Verification items for the finished model (mm, model axes). A direction names the side the tool comes from. Coordinates: 2 decimals unless noted, no trailing zeros. Write each loop counter-clockwise with the first axis right and the second up, starting at its lowest first coordinate (ties: lowest second). Pieces come first, ordered by that corner, then holes.
```python
from build123d import *

# Parameters (mm, degrees)
SKETCH1_R           = 63.5
SKETCH1_R_2         = 3.96875
BOSS_EXTRUDE1_DEPTH = 12.7
SKETCH2_R           = 53.34
SKETCH2_R_2         = 12.7
CUT_EXTRUDE1_DEPTH  = 10.16


with BuildPart() as part:
    # Sketch1 → Boss-Extrude1 (new body, symmetric)
    with BuildSketch(Plane.XY):
        Circle(SKETCH1_R)
        Circle(SKETCH1_R_2, mode=Mode.SUBTRACT)
    extrude(amount=BOSS_EXTRUDE1_DEPTH, both=True)

    # Sketch2 → Cut-Extrude1 (cut)
    with BuildSketch(Plane.XY.offset(12.7)):
        Circle(SKETCH2_R)
        Circle(SKETCH2_R_2, mode=Mode.SUBTRACT)
    cut_extrude1 = extrude(amount=-CUT_EXTRUDE1_DEPTH, mode=Mode.SUBTRACT)

    # Mirror1: Cut-Extrude1 across plane
    add(cut_extrude1.mirror(Plane.XY), mode=Mode.SUBTRACT)


solid = part.part
```
1. Sectioned sample at C-C, the plane z = -6.5. Record the boundary of the cut face in (x, y), and give its area (3 significant figures).
2. Draft check along X on faces 4 (the cylindrical face through (-13.77, -61.99, 0.18)), 5 (the cylindrical face through (-0.86, -3.874, -0.178)), 6 (the flat face through (3, 3, 12.7)), 7 (the cylindrical face through (-2.75, -12.4, 7.69)). Enter one of: pulls with the +X half, pulls with the -X half, needs draft (parallel to the pull), parting line crosses it, or undercut.
3. Tool access check on faces 1 (the cylindrical face through (-6.944, 52.886, 7.691)), 2 (the cylindrical face through (-6.944, 52.886, -7.691)), 3 (the flat face through (-14, 52, -12.7)). Record the directions out of +Z, -Z, +X, -X, +Y, -Y that give a thin tool (end or side, any length) a straight path to the whole face; none if there is none.
4. Gauge pin test, flat ends, axial feed: P1, Ø5, axis at x = -33, y = -35, coming from the +Z side; P2, Ø2, axis at y = -10, z = -7, coming from the -X side; P3, Ø2, axis at x = 19.5, z = 8.5, coming from the +Y side. Record the tip position at first contact, or that the pin passes through.
5. Sectioned sample at D-D, the plane y = 25. Record the boundary of the cut face in (x, z).
6. Sectioned sample at A-A, the plane y = 0. Record the boundary of the cut face in (x, z), and give its area (3 significant figures).
7. Material ranges on L1, parallel to Y at x = 0, z = 4; L2, parallel to Z at x = 29, y = -26; L3, parallel to X at y = -6.5, z = 11, recorded low to high.
Outcome:
1. outline: circle Ø127 at (0, 0); circle Ø25.4 at (0, 0); hole circle Ø106.68 at (0, 0); hole circle Ø7.94 at (0, 0)
1. area: 4,190 mm2
2. face 4: parting line crosses it
2. face 5: undercut
2. face 6: needs draft
2. face 7: undercut
3. face 1: +Z
3. face 2: -Z
3. face 3: -Z, +X, -X, +Y, -Y
4. P1: stops at z = 2.54
4. P2: stops at x = -62.86
4. P3: stops at y = 60.75
5. outline: (-58.37, -12.7) - (-47.12, -12.7) - (-47.12, -2.54) - (47.12, -2.54) - (47.12, -12.7) - (58.37, -12.7) - (58.37, 12.7) - (47.12, 12.7) - (47.12, 2.54) - (-47.12, 2.54) - (-47.12, 12.7) - (-58.37, 12.7) - close
6. outline: (-63.5, -12.7) - (-53.34, -12.7) - (-53.34, -2.54) - (-12.7, -2.54) - (-12.7, -12.7) - (-3.97, -12.7) - (-3.97, 12.7) - (-12.7, 12.7) - (-12.7, 2.54) - (-53.34, 2.54) - (-53.34, 12.7) - (-63.5, 12.7) - close; (3.97, -12.7) - (12.7, -12.7) - (12.7, -2.54) - (53.34, -2.54) - (53.34, -12.7) - (63.5, -12.7) - (63.5, 12.7) - (53.34, 12.7) - (53.34, 2.54) - (12.7, 2.54) - (12.7, 12.7) - (3.97, 12.7) - close
6. area: 1,370 mm2
7. L1: y = -63.5 to -53.34, -12.7 to -3.97, 3.97 to 12.7, 53.34 to 63.5
7. L2: z = -2.54 to 2.54
7. L3: x = -63.17 to -52.94, -10.91 to 10.91, 52.94 to 63.17
